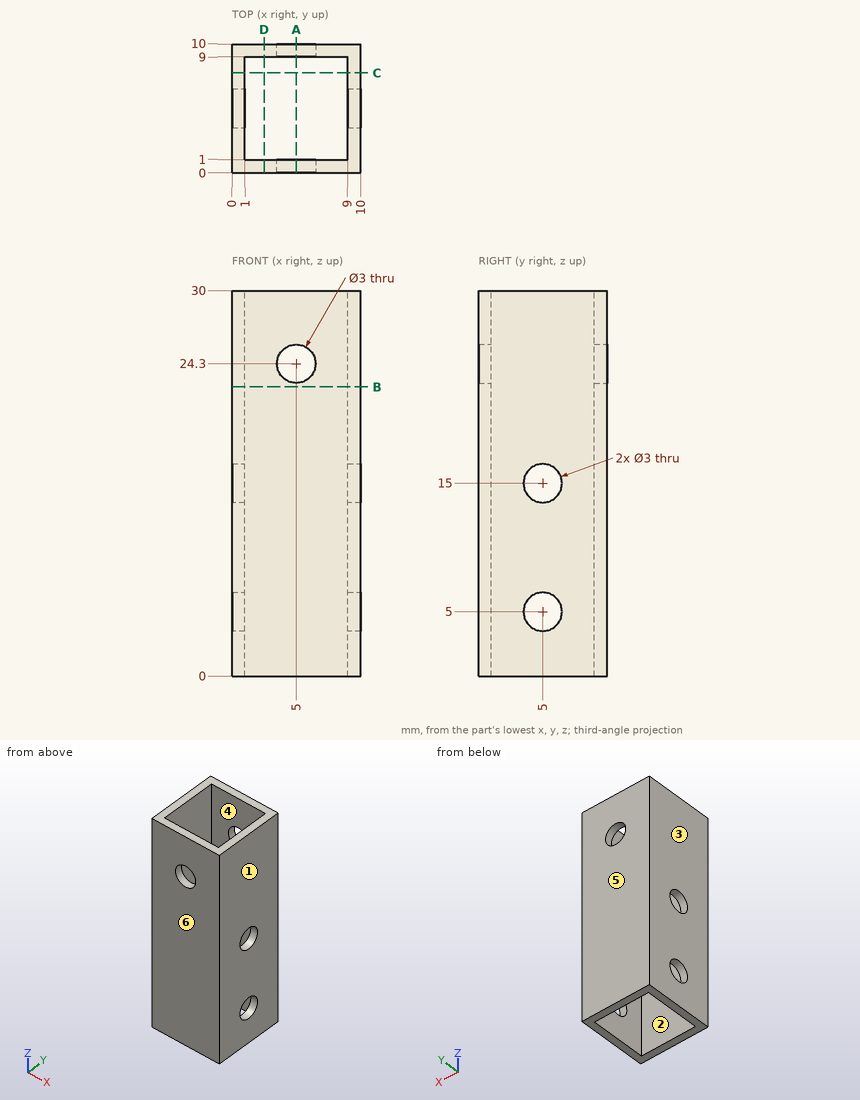
Verification items for this drawing (mm, ordinates from the low corner). A direction names the side the tool comes from. Coordinates: 2 decimals unless noted, no trailing zeros. Loops run counter-clockwise (first coordinate to the right, second up) from the corner with the lowest first, then second, coordinate; pieces in that order, holes last. Notation, with made-up numbers: (54.5, 62) - (79.5, 62) arc R23 cw to (79.5, 96) - close; hole circle Ø9 at (10, 32). An arc over 180 degrees is marked (long way). One line per item, written item: value. Start each with the question number.
(1) Material ranges on line 1 (X direction, y = 6.75, z = 25); line 2 (Z direction, x = 0.5, y = 5.25), recorded low to high. Write a range as [from, to].
(2) Depth check by flat-ended pin: P1, Ø1.8, axis at x = 5, z = 24.3, coming from the +Y side. Enter the tip coordinate at first touch or a pass-through.
(3) Mould release check, pull along Y, two halves, no side actions. Record for the marked faces 3, 4, 5 and 6: released by +Y, released by -Y, zero draft, split by the parting line, or undercut.
(4) Tool access check on the marked faces 1 and 2. Record the directions out of +Z, -Z, +X, -X, +Y, -Y that give a thin tool (end or side, any length) a straight path to the whole face; none if there is none.
(5) Cross-section at A-A on x = 5. Enter the section's corners in (y, z), plus the area to 3 significant figures.
(6) Cross-section at B-B on z = 22.5. Enter the section's corners in (x, y), plus the area to 3 significant figures.
(7) Cross-section at C-C on y = 7.75. Enter the section's corners in (x, z).
Results below:
1. line 1: x = [0, 1], [9, 10]
1. line 2: z = [0, 3.52], [6.48, 13.52], [16.48, 30]
2. P1: passes through
3. face 3: zero draft
3. face 4: undercut
3. face 5: released by +Y
3. face 6: released by -Y
4. face 1: +Z, -Z, +X, +Y, -Y
4. face 2: +Z, -Z
5. outline: (0, 0) - (1, 0) - (1, 22.8) - (0, 22.8) - close; (0, 25.8) - (1, 25.8) - (1, 30) - (0, 30) - close; (9, 0) - (10, 0) - (10, 22.8) - (9, 22.8) - close; (9, 25.8) - (10, 25.8) - (10, 30) - (9, 30) - close
5. area: 54.0 mm2
6. outline: (0, 0) - (10, 0) - (10, 10) - (0, 10) - close; hole (1, 1) - (9, 1) - (9, 9) - (1, 9) - close
6. area: 36.0 mm2
7. outline: (0, 0) - (1, 0) - (1, 30) - (0, 30) - close; (9, 0) - (10, 0) - (10, 30) - (9, 30) - close
